Input: dimensioned drawing with shaded views. Units: mm. Origin: part minimum x, y, z. A direction names the side the tool comes from. Round coordinates to 2 decimals unless told otherwise and drop trailing zeros. Order: outer loops, then holes, each group sorted by start corner. A loop starts at its lowest first (then second) coordinate and runs counter-clockwise, first axis right, second up. Notation, with made-up numbers: M 85.5,20.25 L 135.5,20.25 A25 cw 135.5,49.25 Z; hole C 0,-38 d8. An arc over 180 degrees is marked long. One line per question, with ' | ' between items.
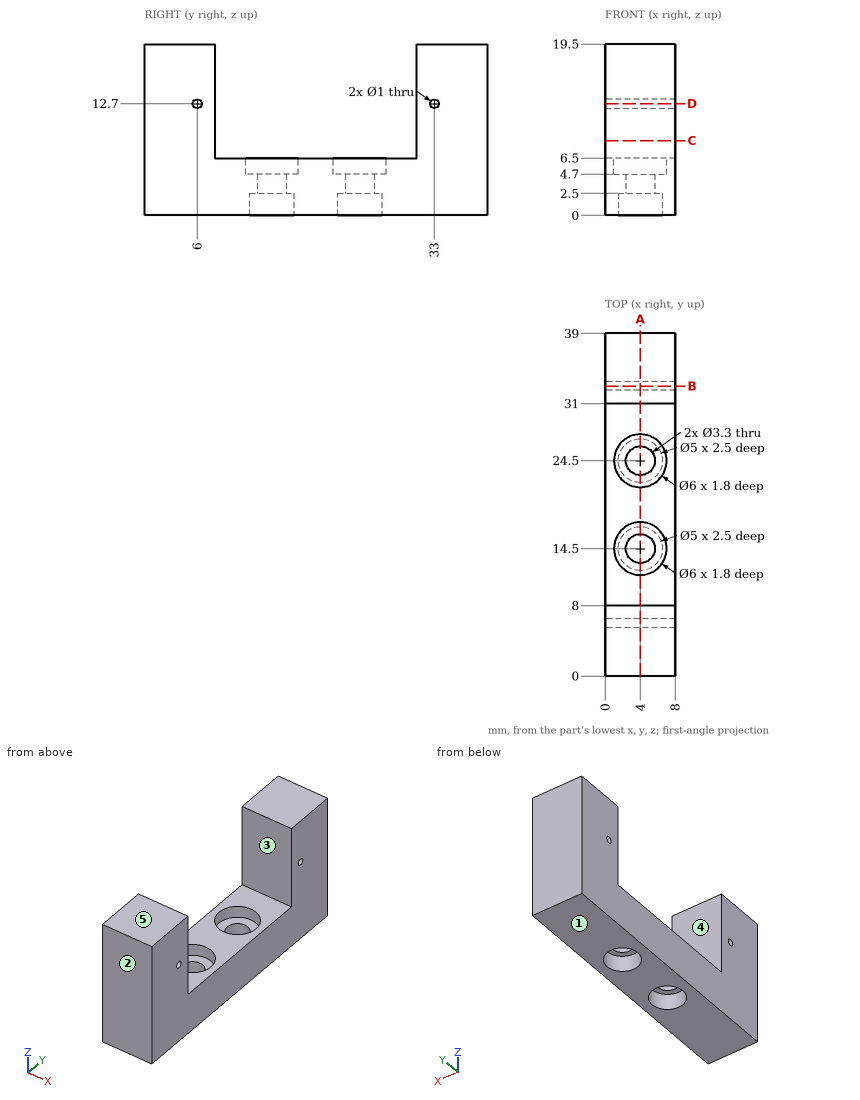
Item 1: Section query C-C, the plane z = 8.5. Return loops of the section in (x, y), plus the area to 3 significant figures.
Report:
outline: M 0,0 L 8,0 L 8,8 L 0,8 Z; M 0,31 L 8,31 L 8,39 L 0,39 Z | area: 128 mm²
Item 2: Line query: line 1 along Y through (x, z) = (2.25, 12.7); line 2 along X through (y, z) = (14.5, 0.95); line 3 along Y through (x, z) = (2.75, 5). Output: solid intervals per line, ascending. Write a range as from..to.
Report:
line 1: 0..5.5, 6.5..8, 31..32.5, 33.5..39 | line 2: 0..1.5, 6.5..8 | line 3: 0..11.77, 17.23..21.77, 27.23..39
Item 3: First-contact query: pin 1 (3.5 mm diameter, centred on x = 4, y = 24.5, fed in from -Z); pin 2 (2.5 mm diameter, centred on x = 4, y = 24.5, fed in from +Z); pin 3 (1.5 mm diameter, centred on x = 6, y = 17, fed in from +Z); pin 4 (4 mm diameter, centred on x = 4, y = 14.5, fed in from +Z). Flat tips, straight axial feed; report the tip coordinate or a pass-through.
Report:
pin 1: z = 2.5 | pin 2: through | pin 3: z = 6.5 | pin 4: z = 4.7
Item 4: Mould query, pull axis Y, two halves, no side actions, for the marked faces 1, 2 and 3. Classes: +Y half, -Y half, draft (parallel to the pull), parting line (faces both ways), or undercut.
Report:
face 1: draft | face 2: -Y half | face 3: undercut
Item 5: Access query for the marked faces 4 and 5. Directions: +Z, -Z, +X, -X, +Y, -Y. A direction counts if a zero-diameter tool reaches every point of the face in a straight line with its end or side. Return the directions, or none.
Report:
face 4: +Z, +X, -X | face 5: +Z, +X, -X, +Y, -Y
Item 6: Section query B-B, the plane y = 33. Return loops of the section in (x, z), plus the area to 3 significant figures.
Report:
outline: M 0,0 L 8,0 L 8,12.2 L 0,12.2 Z; M 0,13.2 L 8,13.2 L 8,19.5 L 0,19.5 Z | area: 148 mm²
Item 7: Section query D-D, the plane z = 12.7. Return loops of the section in (x, y).
Report:
outline: M 0,0 L 8,0 L 8,5.5 L 0,5.5 Z; M 0,6.5 L 8,6.5 L 8,8 L 0,8 Z; M 0,31 L 8,31 L 8,32.5 L 0,32.5 Z; M 0,33.5 L 8,33.5 L 8,39 L 0,39 Z
Item 8: Section query A-A, the plane x = 4. Give the number of separate pieces and of enclosed holes in the cut face, plus the area to 3 significant figures.
Report:
separate pieces: 3 | enclosed holes: 2 | area: 399 mm²
